Autodesk Fusion 360 part; units mm, degrees
sketch "Sketch1" plane through (0, 0, 0) normal (0, 0, 1) x (1, 0, 0)
  line L0 (5, 0) -> (145, 0)
  line L1 (150, 5) -> (150, 85)
  line L2 (145, 90) -> (5, 90)
  line L3 (0, 85) -> (0, 5)
  line L4 (123.8126, 41.439) -> (63.8126, 41.439)
  line L5 (63.8126, 41.439) -> (63.8126, 72.439)
  line L6 (63.8126, 72.439) -> (123.8126, 72.439)
  line L7 (123.8126, 72.439) -> (123.8126, 41.439)
  line L8 (123.8126, 41.439) -> (63.8126, 72.439) construction
  line L9 (63.8126, 41.439) -> (123.8126, 72.439) construction
  line L10 (138.8126, 36.439) -> (48.8126, 36.439)
  line L11 (48.8126, 36.439) -> (48.8126, 77.439)
  line L12 (48.8126, 77.439) -> (138.8126, 77.439)
  line L13 (138.8126, 77.439) -> (138.8126, 36.439)
  line L14 (138.8126, 36.439) -> (48.8126, 77.439) construction
  line L15 (48.8126, 36.439) -> (138.8126, 77.439) construction
  line L16 (35.5073, 47.439) -> (13.5073, 47.439)
  line L17 (13.5073, 47.439) -> (13.5073, 77.439)
  line L18 (13.5073, 77.439) -> (35.5073, 77.439)
  line L19 (35.5073, 77.439) -> (35.5073, 47.439)
  line L20 (35.5073, 47.439) -> (13.5073, 77.439) construction
  line L21 (13.5073, 47.439) -> (35.5073, 77.439) construction
  circle A0 centre (24.5073, 20.2167) radius 3.5
  circle A1 centre (93.8126, 20.2167) radius 10.5
  arc A2 (5, 90) -> (0, 85) centre (5, 85) ccw
  arc A3 (150, 85) -> (145, 90) centre (145, 85) ccw
  arc A4 (145, 0) -> (150, 5) centre (145, 5) ccw
  arc A5 (0, 5) -> (5, 0) centre (5, 5) ccw
  circle A6 centre (5, 85) radius 1.5
  circle A7 centre (145, 85) radius 1.5
  circle A8 centre (145, 5) radius 1.5
  circle A9 centre (5, 5) radius 1.5
  point P0 (150, 0)
  point P1 (0, 90)
  point P2 (93.8126, 56.939)
  point P3 (93.8126, 56.939)
  point P4 (24.5073, 62.439)
  dimension "d1" = 150
  dimension "d2" = 90
  dimension "d3" = 60
  dimension "d4" = 31
  dimension "d5" = 90
  dimension "d6" = 41
  dimension "d7" = 22
  dimension "d8" = 30
  dimension "d9" = 7
  dimension "d10" = 21
  dimension "d13" = 5
  dimension "d14" = 5
  dimension "d15" = 5
  dimension "d16" = 5
  dimension "d17" = 3
  dimension "d18" = 3
  dimension "d19" = 3
  dimension "d20" = 3
extrude "Extrude3" add sketch "Sketch1" along normal blind 3 contours L0 L1 L2 L3 A2 A3 A4 A5 | L10 L11 L12 L13
fillet "Fillet1" radius 2 4 edges at (3.6015, 85.5424, 3) (143.6015, 85.5424, 3) (143.6015, 5.5424, 3) (3.6015, 5.5424, 3)
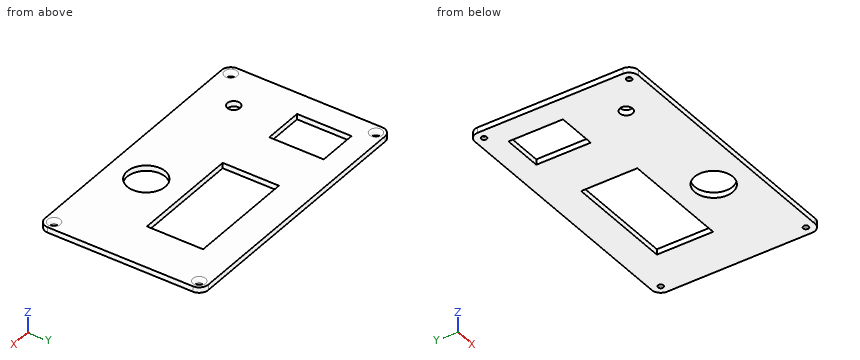
Can you work these out from the model? Positions are in its coordinate system, mm. Give positions to 0.01 mm unless a question says otherwise; leave off trailing zeros. Loops run counter-clockwise (first coordinate to the right, second up) from the corner with the lowest first, then second, coordinate; pieces in that order, holes last. Notation, with made-up numbers: (10, 29) -> (15, 29) arc R24 cw to (15, 62) -> close; hole circle Ø2 at (63, 65.5). An arc over 180 degrees is marked (long way). Use one line per item in the form item = value.
1) If we section it at A-A (y = 66.5): Please give me the cut outline in (x, z), plus the area to 3 significant figures.
Answers:
outline = (0, 0) -> (13.51, 0) -> (13.51, 3) -> (0, 3) -> close; (35.51, 0) -> (63.81, 0) -> (63.81, 3) -> (35.51, 3) -> close; (123.81, 0) -> (150, 0) -> (150, 3) -> (123.81, 3) -> close
area = 204 mm²
2) If we section it at D-D (z = 2.3): Count the separate pieces of the cut face and the enclosed holes in it, plus the area to 3 significant figures.
Answers:
separate_pieces = 1
enclosed_holes = 8
area = 10,500 mm²
3) If we section it at B-B (x = 79): Please give me the cut outline in (y, z), plus the area to 3 significant figures.
Answers:
outline = (0, 0) -> (41.44, 0) -> (41.44, 3) -> (0, 3) -> close; (72.44, 0) -> (90, 0) -> (90, 3) -> (72.44, 3) -> close
area = 177 mm²
4) I need wall thicknesses on line 1 along Y through (x, z) = (5, 0.65); line 2 along Y through (x, z) = (94, 1.1); line 3 along Y through (x, z) = (65, 2.9). Which ranges of each line are inside material? Lowest first, please.
Answers:
line_1 = 0 to 3.5, 6.5 to 83.5, 86.5 to 90
line_2 = 0 to 9.72, 30.72 to 41.44, 72.44 to 90
line_3 = 0 to 41.44, 72.44 to 90
5) If we section it at C-C (y = 27.5): Please give me the cut outline in (x, z), plus the area to 3 significant figures.
Answers:
outline = (0, 0) -> (86.25, 0) -> (86.25, 3) -> (0, 3) -> close; (101.38, 0) -> (150, 0) -> (150, 3) -> (101.38, 3) -> close
area = 405 mm²
